Geometry check sheet. Reference: the model listing, model coordinates, mm. A direction names the side the tool comes from. Coordinates: 2 decimals unless noted, no trailing zeros. Write each loop counter-clockwise with the first axis right and the second up, starting at its lowest first coordinate (ties: lowest second). Pieces come first, ordered by that corner, then holes. Notation, with made-up numbers: (-16.75, 77.25) - (25.25, 77.25) arc R14 cw to (25.25, 103.25) - close; hole circle Ø3 at (-18.5, -36.5). An arc over 180 degrees is marked (long way). Answer as a JSON object with one key per item and string values. Group by question number.
from build123d import *

# Parameters (mm, degrees)
F1_DEPTH      = 206.375
F2_W          = 19.05
F2_H          = 4.7625
F3_DEPTH      = 9.526
F3_DEPTH_BACK = 9.526


with BuildPart() as f1:
    # F0 (on Front) → F1 (new body, symmetric)
    with BuildSketch(Plane.XZ):
        Polygon((9.525, 7.9375), (-9.525, 7.9375), (-9.525, -7.9375), (9.525, -7.9375), (9.525, -3.175), (3.175, -3.175), (3.175, 3.175), (9.525, 3.175), align=None)
    extrude(amount=F1_DEPTH, both=True)

    # F2 (on Right) → F3 (cut, two sides)
    with BuildSketch(Plane.YZ) as f3_sk:
        with Locations((-196.85, 5.55625)):
            Rectangle(F2_W, F2_H)
        with Locations((-196.85, -5.55625)):
            Rectangle(F2_W, F2_H)
        with Locations((196.85, 5.55625)):
            Rectangle(F2_W, F2_H)
        with Locations((196.85, -5.55625)):
            Rectangle(F2_W, F2_H)
        with Locations((0, 5.55625)):
            Rectangle(F2_W, F2_H)
    extrude(amount=-F3_DEPTH, mode=Mode.SUBTRACT)
    extrude(f3_sk.sketch, amount=F3_DEPTH_BACK, mode=Mode.SUBTRACT)


solid = f1.part
(1) Draft check along Z on faces 1 (the face through (0, -100, 7.938)), 2 (the face through (-3, -206.375, 0)), 3 (the face through (-3, -197, -3.175)), 4 (the face through (3.175, -3, 0)). Enter one of: +Z half, -Z half, draft (parallel to the pull), parting line (faces both ways), or undercut.
(2) Set-up check for faces 5 (the face through (-3, 0, 3.175)), 6 (the face through (6, -100, 3.175)), 7 (the face through (-3, 197, -3.175)): record each of +Z, -Z, +X, -X, +Y, -Y from which the full face is reachable in a straight line by a thin tool's end or side.
(3) Section check A-A (x = 6.25). Record the cut outline in (y, z) (1 decimal).
(4) Section check B-B (y = -79.5). Record the cut outline in (x, z) (1 decimal).
(5) Section check C-C (z = 0.5). Record the cut outline in (x, y) (3 decimals), and give its area (3 significant figures).
(6) Material ranges on L1, parallel to Z at x = 6.75, y = 118.5 (1 decimal); L2, parallel to X at y = -58, z = -0.5 (3 decimals); L3, parallel to Y at x = 1.75, z = -5.25 (3 decimals), recorded low to high. Write a range as [from, to].
(7) Gauge pin test, flat ends, axial feed: pin 1 (10 mm diameter, centred on x = -0.5, y = 192.5, fed in from +Z) (3 decimals); pin 2 (10 mm diameter, centred on x = 0, y = -200.5, fed in from -Z) (3 decimals); pin 3 (2.5 mm diameter, centred on x = 0.5, z = 6.5, fed in from +Y) (3 decimals). Record the tip position at first contact, or that the pin passes through.
Conclusion:
{
 "1": {"face 1": "+Z half", "face 2": "draft", "face 3": "-Z half", "face 4": "undercut"},
 "2": {"face 5": "+Z, +X, -X", "face 6": "+X, +Y, -Y", "face 7": "-Z, +X, -X, +Y"},
 "3": {"outline": "(-187.3, -7.9) - (187.3, -7.9) - (187.3, -3.2) - (-187.3, -3.2) - close; (-187.3, 3.2) - (-9.5, 3.2) - (-9.5, 7.9) - (-187.3, 7.9) - close; (9.5, 3.2) - (187.3, 3.2) - (187.3, 7.9) - (9.5, 7.9) - close"},
 "4": {"outline": "(-9.5, -7.9) - (9.5, -7.9) - (9.5, -3.2) - (3.2, -3.2) - (3.2, 3.2) - (9.5, 3.2) - (9.5, 7.9) - (-9.5, 7.9) - close"},
 "5": {"outline": "(-9.525, -206.375) - (3.175, -206.375) - (3.175, 206.375) - (-9.525, 206.375) - close", "area": "5,240 mm^2"},
 "6": {"L1": "z = [-7.9, -3.2], [3.2, 7.9]", "L2": "x = [-9.525, 3.175]", "L3": "y = [-187.325, 187.325]"},
 "7": {"pin 1": "stops at z = 3.175", "pin 2": "stops at z = -3.175", "pin 3": "stops at y = 187.325"}
}
